Work out the finished part from the listing and answer in its coordinate system (mm). Face numbers are marked on the shaded views. A direction names the side the tool comes from. Give positions to 0.01 mm unless a question says otherwise; leave off trailing zeros. Loops run counter-clockwise (first coordinate to the right, second up) from the corner with the lowest first, then second, coordinate; pieces in that order, holes last. Notation, with made-up numbers: M 56.5,35.25 L 112.5,35.25 A20 ccw 112.5,69.25 Z; hole C 5,-36.75 d9. An arc over 180 degrees is marked long. Use a Markdown table: item, result.
```python
from build123d import *

# Parameters (mm, degrees)
SKETCH1_W           = 13
SKETCH1_H           = 30
BOSS_EXTRUDE1_DEPTH = 15
SKETCH2_R           = 1
BOSS_EXTRUDE2_DEPTH = 7.5
SKETCH3_R           = 3
BOSS_EXTRUDE3_DEPTH = 6
BOSS_EXTRUDE4_START = 17.5
SKETCH4_R           = 3
BOSS_EXTRUDE4_DEPTH = 17.5
SKETCH5_R           = 1
CUT_EXTRUDE1_DEPTH  = 38.033768374
SKETCH6_W           = 1.5
SKETCH6_H           = 8
CUT_EXTRUDE2_DEPTH  = 35.767082226


with BuildPart() as part:
    # Sketch1 → Boss-Extrude1 (new body)
    with BuildSketch(Plane.XY):
        Rectangle(SKETCH1_W, SKETCH1_H)
    extrude(amount=BOSS_EXTRUDE1_DEPTH)

    # Sketch2 → Boss-Extrude2 (add)
    with BuildSketch(Plane(origin=(0, 15, 0), x_dir=(1, 0, 0), z_dir=(0, 1, 0))):
        with Locations(Location((0, -7.5, 0), (0, 0, 90))):
            Circle(SKETCH2_R)
    extrude(amount=BOSS_EXTRUDE2_DEPTH)

    # Sketch3 → Boss-Extrude3 (add)
    with BuildSketch(Plane(origin=(0, 22.5, 0), x_dir=(1, 0, 0), z_dir=(0, 1, 0))):
        with Locations(Location((0, -7.5, 0), (0, 0, 270))):
            Circle(SKETCH3_R)
    extrude(amount=BOSS_EXTRUDE3_DEPTH)

    # Sketch4 → Boss-Extrude4 (add)
    with BuildSketch(Plane.XZ.offset(15).offset(BOSS_EXTRUDE4_START)):
        with Locations(Location((0, 7.5, 0), (0, 0, 90))):
            Circle(SKETCH4_R)
    extrude(amount=-BOSS_EXTRUDE4_DEPTH)

    # Sketch5 → Cut-Extrude1 (cut, through all)
    with BuildSketch(Plane(origin=(3, 0, 0), x_dir=(0, 0, -1), z_dir=(1, 0, 0))):
        with Locations((-7.5, -29.5)):
            Circle(SKETCH5_R)
    extrude(amount=-CUT_EXTRUDE1_DEPTH, mode=Mode.SUBTRACT)

    # Sketch6 → Cut-Extrude2 (cut, through all)
    with BuildSketch(Plane(origin=(0, 0, 4.5), x_dir=(-1, 0, 0), z_dir=(0, 0, -1))):
        with Locations((0, -28.5)):
            Rectangle(SKETCH6_W, SKETCH6_H)
    extrude(amount=-CUT_EXTRUDE2_DEPTH, mode=Mode.SUBTRACT)


solid = part.part
```
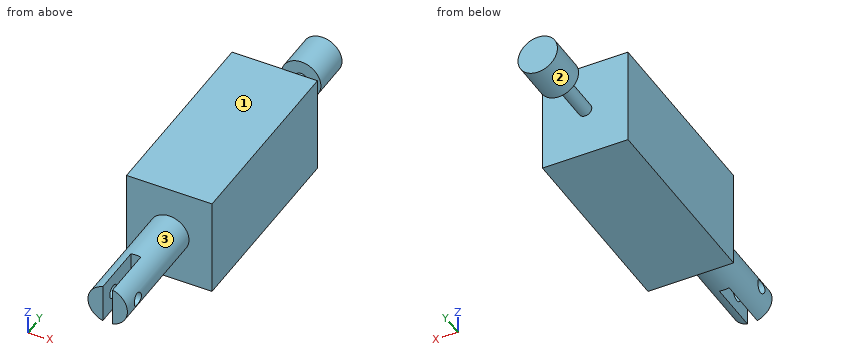
(1) A cutting plane is placed at B-B (x = -2.25). Write down the section's boundary in (y, z).
Entries:
| item | result |
|---|---|
| outline | M -32.5,5.52 L -15,5.52 L -15,0 L 15,0 L 15,15 L -15,15 L -15,9.48 L -32.5,9.48 Z; M 22.5,5.52 L 28.5,5.52 L 28.5,9.48 L 22.5,9.48 Z; hole C -29.5,7.5 d2 |
(2) A cutting plane is placed at A-A (z = 7.5). Write down the section's boundary in (x, y).
Entries:
| item | result |
|---|---|
| outline | M -6.5,-15 L -3,-15 L -3,-28.5 L -0.75,-28.5 L -0.75,-24.5 L 0.75,-24.5 L 0.75,-28.5 L 3,-28.5 L 3,-15 L 6.5,-15 L 6.5,15 L 1,15 L 1,22.5 L 3,22.5 L 3,28.5 L -3,28.5 L -3,22.5 L -1,22.5 L -1,15 L -6.5,15 Z; M -3,-32.5 L -0.75,-32.5 L -0.75,-30.5 L -3,-30.5 Z; M 0.75,-32.5 L 3,-32.5 L 3,-30.5 L 0.75,-30.5 Z |
(3) Consider probe 1 along Y at (x, z) = (1.9, 7.5); probe 2 along Y at (x, z) = (1, 10); probe 3 along Y at (x, z) = (-0.5, 5.5). Determine where each line is inside the solid, lowest interval first. Write a range as [from, to].
Entries:
| item | result |
|---|---|
| probe 1 | y = [-32.5, -30.5], [-28.5, 15], [22.5, 28.5] |
| probe 2 | y = [-32.5, 15], [22.5, 28.5] |
| probe 3 | y = [-24.5, 15], [22.5, 28.5] |
(4) Which of the six approach directions +Z, -Z, +X, -X, +Y, -Y give full straight-line access (tool end or side, diameter ignored) to the marked faces 1, 2 and 3?
Entries:
| item | result |
|---|---|
| face 1 | +Z, +X, -X, +Y, -Y |
| face 2 | +Y |
| face 3 | -Y |
(5) Given P1, Ø4, axis at x = -2.5, y = -24, coming from the +Z side; P2, Ø3, axis at y = -29.5, z = 7.5, coming from the +X side; P3, Ø6.5, axis at y = -29.5, z = 6.5, coming from the -X side; P4, Ø3, axis at x = -4, z = 7.5, coming from the +Y side, each flat-ended and moving along its own axis, determine where each tip first touches the part or whether it passes through.
Entries:
| item | result |
|---|---|
| P1 | stops at z = 10.46 |
| P2 | stops at x = 3 |
| P3 | stops at x = -3 |
| P4 | stops at y = 28.5 |
(6) A cutting plane is placed at C-C (y = -27). Write down the section's boundary in (x, z), and give its area (3 significant figures).
Entries:
| item | result |
|---|---|
| outline | M -0.75,4.6 L -0.75,10.4 A3 ccw Z; M 0.75,4.6 A3 ccw 0.75,10.4 Z |
| area | 19.4 mm² |
(7) A cutting plane is placed at D-D (x = 0). Write down the section's boundary in (y, z), and give its area (3 significant figures).
Entries:
| item | result |
|---|---|
| outline | M -24.5,4.5 L -15,4.5 L -15,0 L 15,0 L 15,6.5 L 22.5,6.5 L 22.5,4.5 L 28.5,4.5 L 28.5,10.5 L 22.5,10.5 L 22.5,8.5 L 15,8.5 L 15,15 L -15,15 L -15,10.5 L -24.5,10.5 Z |
| area | 558 mm² |
